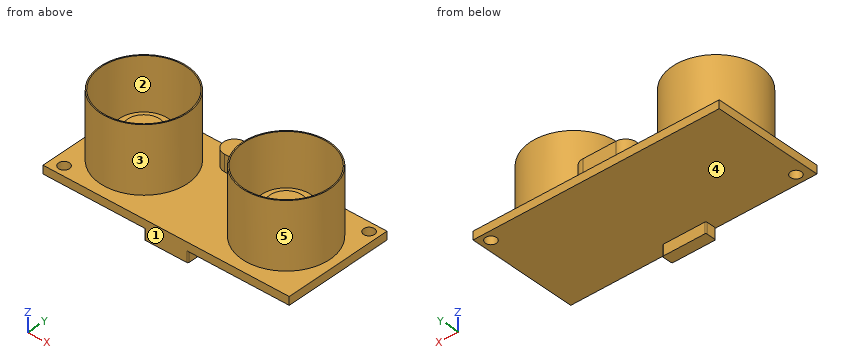
```python
from build123d import *

# Parameters (mm, degrees)
CROQUIS1_W                = 45
CROQUIS1_H                = 20
CROQUIS1_R                = 1
SALIENTE_EXTRUIR1_DEPTH   = 1.5
CROQUIS2_R                = 8
SALIENTE_EXTRUIR2_DEPTH   = 12
CROQUIS4_W                = 2
CROQUIS4_H                = 2
SALIENTE_EXTRUIR4_DEPTH   = 2
REDONDEO3_R               = 0.2
SALIENTE_EXTRUIR6_DEPTH   = 3
VACIADO1_START            = 0.2
VACIADO1_OUTLINE_R        = 7.8
VACIADO1_DEPTH            = 13.1
VACIADO1_2_OUTLINE_W      = 44.6
VACIADO1_2_OUTLINE_H      = 19.6
VACIADO1_2_OUTLINE_R      = 1.2
VACIADO1_2_OUTLINE_R_2    = 7.8
VACIADO1_2_DEPTH          = 1.1
VACIADO1_START_2          = 1.3
VACIADO1_3_DEPTH          = 3
VACIADO1_START_3          = 13.3
VACIADO1_4_OUTLINE_R      = 7.8
VACIADO1_4_DEPTH          = 0.2
VACIADO1_START_4          = -1.8
VACIADO1_5_OUTLINE_W      = 7.6
VACIADO1_5_OUTLINE_H      = 1.6
VACIADO1_5_DEPTH          = 2
CROQUIS9_R                = 4.5
SALIENTE_EXTRUIR8_DEPTH   = 6.15
CROQUIS10_R               = 2.5
SALIENTE_EXTRUIR9_DEPTH   = 0.68
SALIENTE_EXTRUIR9_DRAFT   = -34
CORTAR_EXTRUIR1_START     = -12
CROQUIS12_R               = 7.8
CORTAR_EXTRUIR1_DEPTH     = 12
SIMETR_A3_COPY_1_SKETCH_R = 2.5
SIMETR_A3_COPY_1_DEPTH    = 0.68
SIMETR_A3_COPY_1_DRAFT    = -34


# Read off the part's stored shape, not the designer's step: Vaciado1
with BuildPart() as part:
    # Croquis1 → Saliente-Extruir1 (new body)
    with BuildSketch(Plane.XY):
        with Locations((0, 3.35)):
            Rectangle(CROQUIS1_W, CROQUIS1_H)
        with Locations((20.733115081, 11.657404702)):
            Circle(CROQUIS1_R, mode=Mode.SUBTRACT)
        with Locations((-20.266884919, -4.842595298)):
            Circle(CROQUIS1_R, mode=Mode.SUBTRACT)
    extrude(amount=SALIENTE_EXTRUIR1_DEPTH)

    # Croquis2 → Saliente-Extruir2 (add)
    with BuildSketch(Plane.XY.offset(1.5)):
        with Locations((-13, 3.35)):
            Circle(CROQUIS2_R)
        with Locations(Location((13, 3.35, 0), (0, 0, 180))):
            Circle(CROQUIS2_R)
    extrude(amount=SALIENTE_EXTRUIR2_DEPTH)

    # Croquis4 → Saliente-Extruir4 (add)
    with BuildSketch(Plane(origin=(0, 0, 0), x_dir=(-1, 0, 0), z_dir=(0, 0, -1))):
        with Locations((-3, -5.65)):
            Rectangle(CROQUIS4_W, CROQUIS4_H)
        with Locations((3, -5.65)):
            Rectangle(CROQUIS4_W, CROQUIS4_H)
        with Locations((1, -5.65)):
            Rectangle(CROQUIS4_W, CROQUIS4_H)
        with Locations((-1, -5.65)):
            Rectangle(CROQUIS4_W, CROQUIS4_H)
    extrude(amount=SALIENTE_EXTRUIR4_DEPTH)

    # Redondeo3
    redondeo3_edges = [part.edges().sort_by_distance(p)[0] for p in [
        (-4, -4.65, -1),
        (4, -4.65, -1),
        (4, -6.65, -1),
        (-4, -6.65, -1),
    ]]
    fillet(redondeo3_edges, radius=REDONDEO3_R)

    # Croquis6 → Saliente-Extruir6 (add)
    with BuildSketch(Plane.XY.offset(1.5)):
        with BuildLine():
            Line((-3, 12.689741285), (3, 12.689741285))
            ThreePointArc((3, 12.689741285), (5, 10.689741285), (3, 8.689741285))
            Line((3, 8.689741285), (-3, 8.689741285))
            ThreePointArc((-3, 8.689741285), (-5, 10.689741285), (-3, 12.689741285))
        make_face()
    extrude(amount=SALIENTE_EXTRUIR6_DEPTH)

    # Vaciado1 outline → Vaciado1 (cut)
    with BuildSketch(Plane.XY.offset(VACIADO1_START)):
        with Locations((-13, 3.35)):
            Circle(VACIADO1_OUTLINE_R)
        with Locations((13, 3.35)):
            Circle(VACIADO1_OUTLINE_R)
    extrude(amount=VACIADO1_DEPTH, mode=Mode.SUBTRACT)

    # Vaciado1 2 outline → Vaciado1 2 (cut)
    with BuildSketch(Plane.XY.offset(VACIADO1_START)):
        with Locations((0, 3.35)):
            Rectangle(VACIADO1_2_OUTLINE_W, VACIADO1_2_OUTLINE_H)
        with Locations((-20.266884919, -4.842595298)):
            Circle(VACIADO1_2_OUTLINE_R, mode=Mode.SUBTRACT)
        with Locations((-13, 3.35)):
            Circle(VACIADO1_2_OUTLINE_R_2, mode=Mode.SUBTRACT)
        with Locations((13, 3.35)):
            Circle(VACIADO1_2_OUTLINE_R_2, mode=Mode.SUBTRACT)
        with Locations((20.733115081, 11.657404702)):
            Circle(VACIADO1_2_OUTLINE_R, mode=Mode.SUBTRACT)
    extrude(amount=VACIADO1_2_DEPTH, mode=Mode.SUBTRACT)

    # Vaciado1 3 outline → Vaciado1 3 (cut)
    with BuildSketch(Plane.XY.offset(VACIADO1_START_2)):
        with BuildLine():
            ThreePointArc((-3, 12.489741285), (-4.8, 10.689741285), (-3, 8.889741285))
            Line((-3, 8.889741285), (3, 8.889741285))
            ThreePointArc((3, 8.889741285), (4.8, 10.689741285), (3, 12.489741285))
            Line((3, 12.489741285), (-3, 12.489741285))
        make_face()
    extrude(amount=VACIADO1_3_DEPTH, mode=Mode.SUBTRACT)

    # Vaciado1 4 outline → Vaciado1 4 (cut)
    with BuildSketch(Plane.XY.offset(VACIADO1_START_3)):
        with Locations((13, 3.35)):
            Circle(VACIADO1_4_OUTLINE_R)
    extrude(amount=VACIADO1_4_DEPTH, mode=Mode.SUBTRACT)

    # Vaciado1 5 outline → Vaciado1 5 (cut)
    with BuildSketch(Plane.XY.offset(VACIADO1_START_4)):
        with Locations((0, -5.65)):
            Rectangle(VACIADO1_5_OUTLINE_W, VACIADO1_5_OUTLINE_H)
    extrude(amount=VACIADO1_5_DEPTH, mode=Mode.SUBTRACT)

    # Croquis9 → Saliente-Extruir8 (add)
    with BuildSketch(Plane.XY.offset(0.2)):
        with Locations((13, 3.35)):
            Circle(CROQUIS9_R)
    saliente_extruir8 = extrude(amount=SALIENTE_EXTRUIR8_DEPTH)


with BuildPart() as saliente_extruir9_tool:
    # Croquis10 → Saliente-Extruir9 (with draft: the straight prism first)
    with BuildSketch(Plane.XY.offset(6.35)):
        with Locations((13, 3.35)):
            Circle(CROQUIS10_R)
    extrude(amount=SALIENTE_EXTRUIR9_DEPTH)
    # Saliente-Extruir9: the draft: its side faces are tilted about the plane it starts from
    saliente_extruir9_sides = [saliente_extruir9_tool.faces().sort_by_distance(p)[0] for p in [
        (10.5, 3.35, 6.69),
    ]]
    draft(saliente_extruir9_sides, Plane.XY.offset(6.35), SALIENTE_EXTRUIR9_DRAFT)


with BuildPart() as part_1:
    add(part.part)

    # Saliente-Extruir9: add saliente_extruir9_tool
    add(saliente_extruir9_tool.part)

    # Croquis12 → Cortar-Extruir1 (cut)
    with BuildSketch(Plane.XY.offset(13.5).offset(CORTAR_EXTRUIR1_START)):
        with Locations((-13, 3.35)):
            Circle(CROQUIS12_R)
    extrude(amount=CORTAR_EXTRUIR1_DEPTH, mode=Mode.SUBTRACT)

    # Simetría3: Saliente-Extruir8 across plane
    add(saliente_extruir8.mirror(Plane(origin=(0, 0, 0), x_dir=(0, 0, 1), z_dir=(1, 0, 0))))


with BuildPart() as simetr_a3_copy_1_tool:
    # Simetría3 copy 1 sketch → Simetría3 copy 1 (with draft: the straight prism first)
    with BuildSketch(Plane(origin=(0, 0, 6.35), x_dir=(-1, 0, 0), z_dir=(0, 0, 1))):
        with Locations((13, -3.35)):
            Circle(SIMETR_A3_COPY_1_SKETCH_R)
    extrude(amount=SIMETR_A3_COPY_1_DEPTH)
    # Simetría3 copy 1: the draft: its side faces are tilted about the plane it starts from
    simetr_a3_copy_1_sides = [simetr_a3_copy_1_tool.faces().sort_by_distance(p)[0] for p in [
        (-10.5, 3.35, 6.69),
    ]]
    draft(simetr_a3_copy_1_sides, Plane(origin=(0, 0, 6.35), x_dir=(-1, 0, 0), z_dir=(0, 0, 1)), SIMETR_A3_COPY_1_DRAFT)


with BuildPart() as part_2:
    add(part_1.part)

    # Simetría3 copy 1: add simetr_a3_copy_1_tool
    add(simetr_a3_copy_1_tool.part)


solid = part_2.part
```
The model under review builds one solid part; all positions refer to its coordinate system, in mm. Face numbers are marked on the shaded views. A direction names the side the tool comes from. Round coordinates to 2 decimals unless told otherwise and drop trailing zeros. Write each loop counter-clockwise with the first axis right and the second up, starting at its lowest first coordinate (ties: lowest second). Pieces come first, ordered by that corner, then holes.
(1) We need section D-D on x = 6. Give the boundary of the cut face in (y, z).
(2) Mouldability with a two-part tool opening along X and no side actions: class the marked faces 3, 4 and 5 as +X half, -X half, draft (parallel to the pull), parting line (faces both ways), or undercut.
(3) We need section B-B on x = -13. Give the boundary of the cut face in (y, z), and give its area (3 significant figures).
(4) Wall thickness on L1, parallel to Y at x = 13, z = 5.75; L2, parallel to Z at x = 17.5, y = -3.75; L3, parallel to Y at x = 13, z = 9.75: over which ranges is each line inside the solid? List them lowest first.
(5) Insertion check: pin 1 (4 mm diameter, centred on x = -14, z = 7.5, fed in from +Y); pin 2 (4.5 mm diameter, centred on x = -1, y = 10, fed in from +Z); pin 3 (1.8 mm diameter, centred on x = 0, y = -5.5, fed in from +Z). Each pin has a flat end and moves straight along its axis. Give the tip position at first contact, or say it passes through.
(6) We need section C-C on y = -2.75. Give the boundary of the cut face in (x, z), and give its area (3 significant figures).
(7) We need section A-A on z = 9. Give the boundary of the cut face in (x, y), and give its area (3 significant figures).
(8) Machinability: for the marked faces 1 and 2, which of the approach directions +Z, -Z, +X, -X, +Y, -Y give a long, thin tool a straight path to every point of the face, cutting with its end or side? Answer none if there is none.
Findings below:
1. outline: (-6.65, 0) - (13.35, 0) - (13.35, 1.5) - (7.22, 1.5) - (7.22, 13.5) - (6.79, 13.5) - (6.79, 1.3) - (13.15, 1.3) - (13.15, 0.2) - (-6.45, 0.2) - (-6.45, 1.3) - (-0.09, 1.3) - (-0.09, 13.5) - (-0.52, 13.5) - (-0.52, 1.5) - (-6.65, 1.5) - close
2. face 3: undercut
2. face 4: draft
2. face 5: undercut
3. outline: (-6.65, 0) - (13.35, 0) - (13.35, 1.5) - (11.35, 1.5) - (11.35, 13.5) - (11.15, 13.5) - (11.15, 1.3) - (13.15, 1.3) - (13.15, 0.2) - (7.85, 0.2) - (7.85, 6.35) - (5.85, 6.35) - (6.31, 7.03) - (0.39, 7.03) - (0.85, 6.35) - (-1.15, 6.35) - (-1.15, 0.2) - (-6.45, 0.2) - (-6.45, 1.3) - (-4.45, 1.3) - (-4.45, 13.5) - (-4.65, 13.5) - (-4.65, 1.5) - (-6.65, 1.5) - close
3. area: 69.2 mm2
4. L1: y = -4.65 to -4.45, -1.15 to 7.85, 11.15 to 11.35
4. L2: z = 0 to 0.2, 1.3 to 1.5
4. L3: y = -4.65 to -4.45, 11.15 to 11.35
5. pin 1: stops at y = 11.35
5. pin 2: stops at z = 4.5
5. pin 3: stops at z = 1.5
6. outline: (-22.5, 0) - (22.5, 0) - (22.5, 1.5) - (18.18, 1.5) - (18.18, 13.5) - (17.86, 13.5) - (17.86, 1.3) - (22.3, 1.3) - (22.3, 0.2) - (-22.3, 0.2) - (-22.3, 1.3) - (-17.86, 1.3) - (-17.86, 13.5) - (-18.18, 13.5) - (-18.18, 1.5) - (-22.5, 1.5) - close; (-8.14, 1.3) - (8.14, 1.3) - (8.14, 13.5) - (7.82, 13.5) - (7.82, 1.5) - (-7.82, 1.5) - (-7.82, 13.5) - (-8.14, 13.5) - close
6. area: 29.7 mm2
7. outline: circle Ø16 at (-13, 3.35); circle Ø16 at (13, 3.35); hole circle Ø15.6 at (-13, 3.35); hole circle Ø15.6 at (13, 3.35)
7. area: 19.9 mm2
8. face 1: +Z, -Z, +X, -X, -Y
8. face 2: +Z
